The listing builds one solid part. Answer for the finished solid, in the listing's coordinates (mm). A direction names the side the tool comes from. Give positions to 0.01 mm unless a question says otherwise; leave off trailing zeros. Order: outer loops, then holes, each group sorted by start corner. A loop starts at its lowest first (then second) coordinate and runs counter-clockwise, first axis right, second up. Notation, with made-up numbers: (3, 0.5) - (57, 0.5) arc R19 ccw to (57, 30.5) - close; hole circle Ø9 at (16.5, -39.5). An arc over 180 degrees is marked (long way). Use a Markdown table: item, result. Add a question column.
1) Find section B-B, the plane z = 2.5. Determine the outline of the cut face in (x, y), plus the area to 3 significant figures.
2) Find section D-D, the plane y = 1.7. Determine the outline of the cut face in (x, z).
3) Find section C-C, the plane x = 10.45. Determine the outline of the cut face in (y, z).
4) Flat-ended cylindrical pins translate along their axes: pin 1 (4.5 mm diameter, centred on x = 3.5, y = -10.5, fed in from +Z); pin 2 (2 mm diameter, centred on y = -9.5, z = 2.5, fed in from +X); pin 3 (3 mm diameter, centred on x = -4.5, z = 13.5, fed in from +Y); pin 4 (2 mm diameter, centred on x = -10.45, y = -3.65, fed in from -Z). Find the tip coordinate at first contact, or state that the pin passes through.
5) The mould has two halves that part along Y. Classify faces 1 (the face through (-0.2, 12, 0.5)), 2 (the face through (-9.434, -4.071, 0.493)), 3 (the face through (12.5, -0.2, 0.5)): released by +Y, released by -Y, zero draft, split by the parting line, or undercut.
6) For faces 4 (the face through (-1, -10, 3.7)), 5 (the face through (4.51, -3.03, 8)), 6 (the face through (-1, -8, 2)), 7 (the face through (9.8, -10, 2)), 8 (the face through (-10.6, -10, 2)), determine the directions among +Z, -Z, +X, -X, +Y, -Y from which every point of the face is accessible in a straight line to the end or side of a thin tool.
7) Find section A-A, the plane y = 10.05. Determine the outline of the cut face in (x, z), plus the area to 3 significant figures.
8) Straight lines are drawn through the part: line 1 (Y direction, x = 10.45, z = 0.6); line 2 (X direction, y = -3.65, z = 0.85); line 3 (Y direction, x = -8.75, z = 2.25). For each, find the intervals that lie inside material, in ascending order.
from build123d import *

# Parameters (mm, degrees)
ESBO_O1_W                  = 25
ESBO_O1_H                  = 24
RESSALTO_EXTRUS_O1_DEPTH   = 1
ESBO_O2_W                  = 20.4
ESBO_O2_H                  = 4
RESSALTO_EXTRUS_O2_DEPTH   = 2.7
CORTE_EXTRUS_O1_DEPTH      = 18.536818412
CORTE_EXTRUS_O1_DEPTH_BACK = 18.536818412
ESBO_O3_R                  = 1.1
ESBO_O4_R                  = 7
RESSALTO_EXTRUS_O3_DEPTH   = 15.2
CHANFRO1_SIZE              = 1
CHANFRO1_SIZE2             = 1.732050808


with BuildPart() as part:
    # Esboço1 → Ressalto-extrusão1 (new body)
    with BuildSketch(Plane.XY):
        Rectangle(ESBO_O1_W, ESBO_O1_H)
    extrude(amount=RESSALTO_EXTRUS_O1_DEPTH)

    # Esboço2 → Ressalto-extrusão2 (add)
    with BuildSketch(Plane.XY.offset(1)):
        with Locations((-0.4, -10)):
            Rectangle(ESBO_O2_W, ESBO_O2_H)
    extrude(amount=RESSALTO_EXTRUS_O2_DEPTH)

    # Esboço3 → Corte-extrusão1 (cut, two sides: drawn at the far end of the back side and taken through both)
    with BuildSketch(Plane.XY.offset(1).offset(-CORTE_EXTRUS_O1_DEPTH_BACK)):
        with Locations((10.45, 10.05)):
            Circle(ESBO_O3_R)
        with Locations((-10.45, 10.05)):
            Circle(ESBO_O3_R)
        with Locations((10.45, -3.65)):
            Circle(ESBO_O3_R)
        with Locations((-10.45, -3.65)):
            Circle(ESBO_O3_R)
    extrude(amount=CORTE_EXTRUS_O1_DEPTH + CORTE_EXTRUS_O1_DEPTH_BACK, mode=Mode.SUBTRACT)

    # Esboço4 → Ressalto-extrusão3 (add)
    with BuildSketch(Plane.XY.offset(1)):
        with Locations(Location((-0.65, 1.7, 0), (0, 0, 180))):
            Circle(ESBO_O4_R)
    extrude(amount=RESSALTO_EXTRUS_O3_DEPTH)

    # Chanfro1
    chanfro1_edges = [part.edges().sort_by_distance(p)[0] for p in [
        (6.35, 1.7, 16.2),
    ]]
    chanfro1_side = [part.faces().sort_by_distance(p)[0] for p in [
        (6.35, 1.7, 8.6),
    ]]
    chamfer(chanfro1_edges, length=CHANFRO1_SIZE, length2=CHANFRO1_SIZE2, reference=chanfro1_side[0])


solid = part.part
The answers:
| question | item | result |
|---|---|---|
| 1 | outline | (-10.6, -12) - (9.8, -12) - (9.8, -8) - (-10.6, -8) - close; circle Ø14 at (-0.65, 1.7) |
| 1 | area | 236 mm2 |
| 2 | outline | (-12.5, 0) - (12.5, 0) - (12.5, 1) - (6.35, 1) - (6.35, 15.2) - (4.62, 16.2) - (-5.92, 16.2) - (-7.65, 15.2) - (-7.65, 1) - (-12.5, 1) - close |
| 3 | outline | (-12, 0) - (-4.75, 0) - (-4.75, 1) - (-12, 1) - close; (-2.55, 0) - (8.95, 0) - (8.95, 1) - (-2.55, 1) - close; (11.15, 0) - (12, 0) - (12, 1) - (11.15, 1) - close |
| 4 | pin 1 | z = 3.7 |
| 4 | pin 2 | x = 9.8 |
| 4 | pin 3 | y = 8.29 |
| 4 | pin 4 | through |
| 5 | face 1 | released by +Y |
| 5 | face 2 | undercut |
| 5 | face 3 | zero draft |
| 6 | face 4 | +Z, +X, -X, -Y |
| 6 | face 5 | +Z |
| 6 | face 6 | +Z, +X, -X |
| 6 | face 7 | +Z, +X, +Y, -Y |
| 6 | face 8 | +Z, -X, +Y, -Y |
| 7 | outline | (-12.5, 0) - (-11.55, 0) - (-11.55, 1) - (-12.5, 1) - close; (-9.35, 0) - (9.35, 0) - (9.35, 1) - (-9.35, 1) - close; (11.55, 0) - (12.5, 0) - (12.5, 1) - (11.55, 1) - close |
| 7 | area | 20.6 mm2 |
| 8 | line 1 | -12 to -4.75, -2.55 to 8.95, 11.15 to 12 |
| 8 | line 2 | -12.5 to -11.55, -9.35 to 9.35, 11.55 to 12.5 |
| 8 | line 3 | -12 to -8 |
